Input: dimensioned drawing with shaded views. Units: mm. Origin: part minimum x, y, z. Give positions to 0.01 mm unless a question says otherwise; leave off trailing zeros. Order: outer loops, then holes, each group sorted by start corner. A loop starts at its lowest first (then second) coordinate and runs counter-clockwise, first axis right, second up. Notation, with made-up numbers: (14, -3.75) - (69, -3.75) arc R29 ccw to (69, 31.25) - close; hole circle Ø8 at (-5, 16.25). An arc over 180 degrees is marked (long way). Use a Markdown table: item, result.
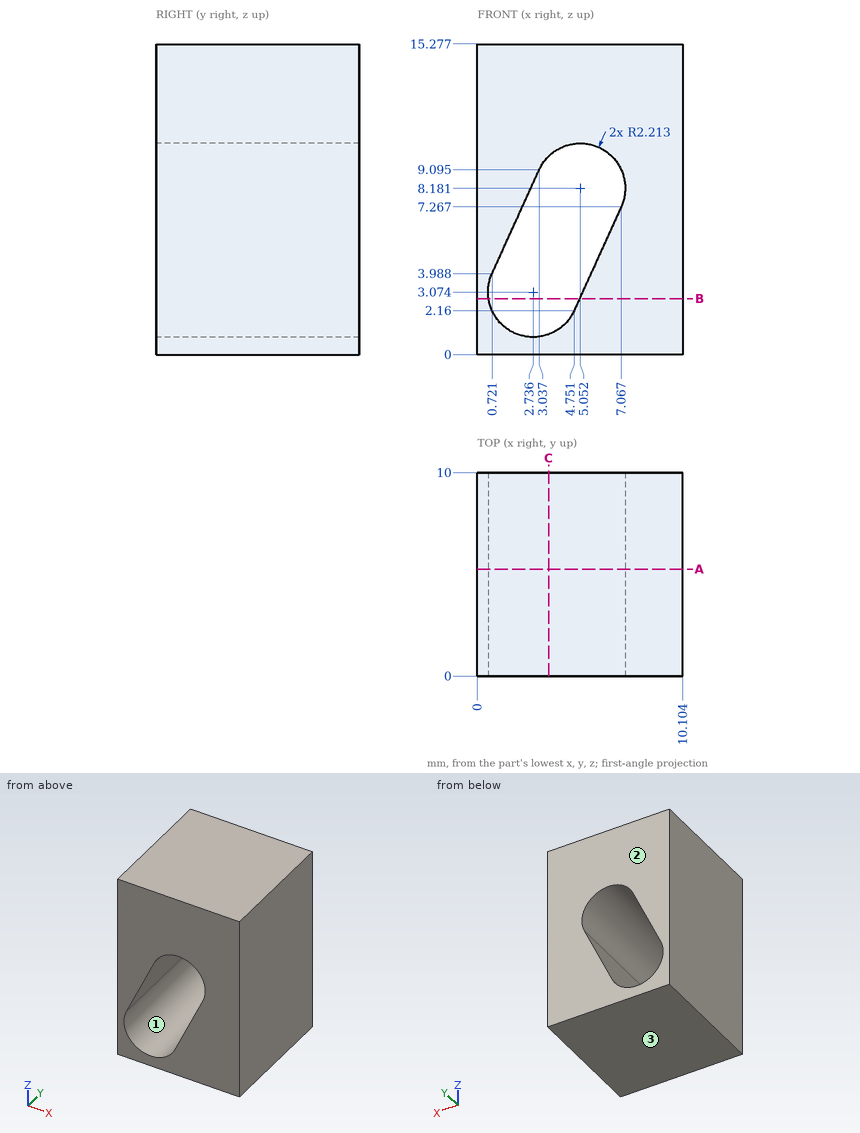
1. Mould query, pull axis Z, two halves, no side actions, for the marked faces 1, 2 and 3. Classes: pulls with the +Z half, pulls with the -Z half, needs draft (parallel to the pull), parting line crosses it, or undercut.
Response:
| item | result |
|---|---|
| face 1 | undercut |
| face 2 | needs draft |
| face 3 | pulls with the -Z half |
2. Pin query (flat end, axial travel): pin 1 (1.5 mm diameter, centred on y = 8.5, z = 10.5, fed in from -X). Return the tip coordinate at first contact, or that it passes through.
Response:
| item | result |
|---|---|
| pin 1 | stops at x = 0 |
3. Section query C-C (x = 3.5). Return loops of the section in (y, z).
Response:
| item | result |
|---|---|
| outline | (0, 0) - (10, 0) - (10, 1) - (0, 1) - close; (0, 9.76) - (10, 9.76) - (10, 15.28) - (0, 15.28) - close |
4. Material intervals for line 1 along Z through (x, y) = (2, 1.25) (1 decimal); line 2 along X through (y, z) = (8, 7.75) (1 decimal); line 3 along Z through (x, y) = (3.5, 7.25) (1 decimal), sorted ascending.
Response:
| item | result |
|---|---|
| line 1 | z = 0 to 1, 6.8 to 15.3 |
| line 2 | x = 0 to 2.4, 7.2 to 10.1 |
| line 3 | z = 0 to 1, 9.8 to 15.3 |
5. Section query A-A (y = 5.25). Return loops of the section in (x, z) (1 decimal).
Response:
| item | result |
|---|---|
| outline | (0, 0) - (10.1, 0) - (10.1, 15.3) - (0, 15.3) - close; hole (0.7, 4) arc R2.2 ccw to (4.8, 2.2) - (7.1, 7.3) arc R2.2 ccw to (3, 9.1) - close |
6. Section query B-B (z = 2.75). Return loops of the section in (x, y).
Response:
| item | result |
|---|---|
| outline | (0, 0) - (0.55, 0) - (0.55, 10) - (0, 10) - close; (5.02, 0) - (10.1, 0) - (10.1, 10) - (5.02, 10) - close |
